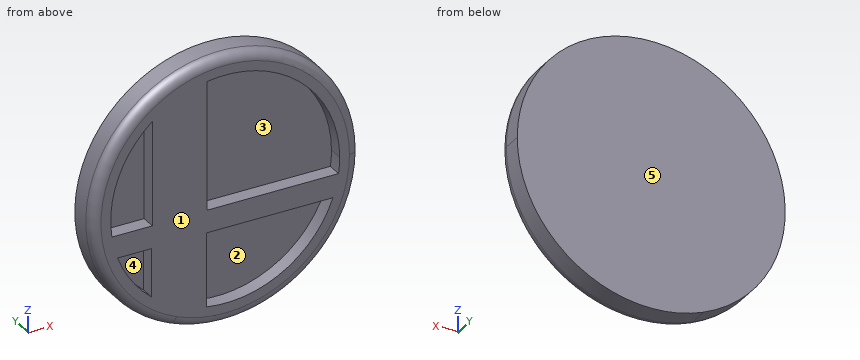
from build123d import *

# Parameters (mm, degrees)
F1_DEPTH = 7.62
F2_DEPTH = 3.81
F3_R     = 2.54


with BuildPart() as f1:
    # F0 (on Front) → F1 (new body)
    with BuildSketch(Plane.XZ):
        with BuildLine():
            ThreePointArc((17.744669, 0), (50.676236, 3.013402), (66.332194, 32.141733))
            ThreePointArc((66.332194, 32.141733), (12.138153, 61.270064), (17.744669, 0))
        make_face()
        with BuildLine():
            ThreePointArc((26.666769, 61.607856), (50.762375, 54.85959), (61.252194, 32.141733))
            ThreePointArc((61.252194, 32.141733), (61.178246, 30.042092), (60.956769, 27.952856))
            ThreePointArc((60.956769, 27.952856), (60.377684, 24.969932), (59.498295, 22.061351))
            ThreePointArc((59.498295, 22.061351), (46.499376, 6.393916), (26.478295, 2.706551))
            ThreePointArc((26.478295, 2.706551), (18.921559, 5.033931), (12.241204, 9.26404))
            ThreePointArc((12.241204, 9.26404), (6.957218, 15.02675), (3.351204, 21.96404))
            ThreePointArc((3.351204, 21.96404), (2.46218, 24.867794), (1.87284, 27.84686))
            ThreePointArc((1.87284, 27.84686), (3.560265, 42.87824), (12.400403, 55.15186))
            ThreePointArc((12.400403, 55.15186), (19.10262, 59.3322), (26.666769, 61.607856))
        make_face(mode=Mode.SUBTRACT)
        with BuildLine():
            Line((26.666769, 27.952856), (26.666769, 61.607856))
            ThreePointArc((26.666769, 61.607856), (19.10262, 59.3322), (12.400403, 55.15186))
            Line((12.400403, 55.15186), (12.400403, 27.84686))
            Line((12.400403, 27.84686), (1.87284, 27.84686))
            ThreePointArc((1.87284, 27.84686), (2.46218, 24.867794), (3.351204, 21.96404))
            Line((3.351204, 21.96404), (12.241204, 21.96404))
            Line((12.241204, 21.96404), (12.241204, 9.26404))
            ThreePointArc((12.241204, 9.26404), (18.921559, 5.033931), (26.478295, 2.706551))
            Line((26.478295, 2.706551), (26.478295, 22.061351))
            Line((26.478295, 22.061351), (59.498295, 22.061351))
            ThreePointArc((59.498295, 22.061351), (60.377684, 24.969932), (60.956769, 27.952856))
            Line((60.956769, 27.952856), (26.666769, 27.952856))
        make_face()
    extrude(amount=F1_DEPTH)

    # F0 (on Front) → F2 (join)
    with BuildSketch(Plane.XZ):
        with BuildLine():
            Line((12.400403, 27.84686), (12.400403, 55.15186))
            ThreePointArc((12.400403, 55.15186), (3.560265, 42.87824), (1.87284, 27.84686))
            Line((1.87284, 27.84686), (12.400403, 27.84686))
        make_face()
        with BuildLine():
            ThreePointArc((60.956769, 27.952856), (61.178246, 30.042092), (61.252194, 32.141733))
            ThreePointArc((61.252194, 32.141733), (50.762375, 54.85959), (26.666769, 61.607856))
            Line((26.666769, 61.607856), (26.666769, 27.952856))
            Line((26.666769, 27.952856), (60.956769, 27.952856))
        make_face()
        with BuildLine():
            ThreePointArc((26.478295, 2.706551), (46.499376, 6.393916), (59.498295, 22.061351))
            Line((59.498295, 22.061351), (26.478295, 22.061351))
            Line((26.478295, 22.061351), (26.478295, 2.706551))
        make_face()
        with BuildLine():
            Line((12.241204, 21.96404), (3.351204, 21.96404))
            ThreePointArc((3.351204, 21.96404), (6.957218, 15.02675), (12.241204, 9.26404))
            Line((12.241204, 9.26404), (12.241204, 21.96404))
        make_face()
    extrude(amount=F2_DEPTH)

    # F3
    f3_edges = [f1.edges().sort_by_distance(p)[0] for p in [
        (45.06972, -7.62, 64.283466),
    ]]
    fillet(f3_edges, radius=F3_R)


solid = f1.part
Model file for the job. Use its own axes, mm. Face numbers are marked on the shaded views. A direction names the side the tool comes from. Coordinates: 2 decimals unless noted, no trailing zeros. Order: outer loops, then holes, each group sorted by start corner. A loop starts at its lowest first (then second) coordinate and runs counter-clockwise, first axis right, second up. Notation, with made-up numbers: M -27,10 L 9,10 A33 ccw 9,39 Z; hole C 33,66 d1. An arc over 180 degrees is marked long. Return JSON: item names as keys, results as strings.
1. Saw through at A-A (y = -6.5). Give the cut face in (x, z) (3 decimals), and give its area (3 significant figures).
Ans:
{"outline": "M 17.914,0.399 A34.491 ccw 65.898,32.142 A34.491 ccw long Z; hole M 1.873,27.847 L 12.4,27.847 L 12.4,55.152 A29.845 ccw Z; hole M 3.351,21.964 A29.845 ccw 12.241,9.264 L 12.241,21.964 Z; hole M 26.478,2.707 A29.845 ccw 59.498,22.061 L 26.478,22.061 Z; hole M 26.667,27.953 L 60.957,27.953 A29.845 ccw 61.252,32.142 A29.845 ccw 26.667,61.608 Z", "area": "1,960 mm^2"}
2. Drill centre lines: probe 1 along Z at (x, y) = (5, -5); probe 2 along X at (y, z) = (-6.25, 52.5); probe 3 along Y at (x, z) = (38, 12). Where is each one in solid material? Low to high.
Ans:
{"probe 1": "9.29 to 18.24, 21.96 to 27.85, 46.05 to 55", "probe 2": "3.38 to 9.58, 12.4 to 26.67, 53.23 to 59.43", "probe 3": "-3.81 to 0"}
3. Saw through at B-B (y = -1). Give the cut face in (x, z) (3 decimals), and give its area (3 significant figures).
Ans:
{"outline": "M 17.745,0 A34.925 ccw 66.332,32.142 A34.925 ccw long Z", "area": "3,830 mm^2"}
4. Flat gauge pins, fed straight in: pin 1 (1.9 mm diameter, centred on y = -5.5, z = 12, fed in from +X); pin 2 (4 mm diameter, centred on x = 47, y = -5.5, fed in from +Z); pin 3 (3 mm diameter, centred on y = -5.5, z = 40, fed in from -X). Where does each tip first touch, or does it go through?
Ans:
{"pin 1": "x = 60.56", "pin 2": "z = 64.3", "pin 3": "x = -2.93"}
5. Pull direction Z, two halves, no side cores. Call the marked faces 1, 2 and 3: +Z half, -Z half, draft (parallel to the pull), parting line (faces both ways), or undercut.
Ans:
{"face 1": "draft", "face 2": "undercut", "face 3": "undercut"}
6. Tool access for the marked faces 4 and 5: list every direction of +Z, -Z, +X, -X, +Y, -Y with a clear straight run to the whole face (end or side of a thin tool).
Ans:
{"face 4": "-Y", "face 5": "+Z, -Z, +X, -X, +Y"}
